from build123d import *

# Parameters (mm, degrees)
SKETCH1_W           = 12.7
SKETCH1_H           = 12.7
BOSS_EXTRUDE1_DEPTH = 2.54
FILLET1_R           = 0.635
SHELL1_START        = 0.635
SHELL1_OUTLINE_W    = 1.905
SHELL1_OUTLINE_H    = 11.43
SHELL1_DEPTH        = 11.43
SKETCH2_R           = 2.54
BOSS_EXTRUDE2_DEPTH = 1.905
BOSS_EXTRUDE3_DEPTH = 0.00254


# Read off the part's stored shape, not the designer's step: Shell1
with BuildPart() as part:
    # Sketch1 → Boss-Extrude1 (new body)
    with BuildSketch(Plane(origin=(0, 0, 0), x_dir=(1, 0, 0), z_dir=(0, 1, 0))):
        with Locations((6.35, 6.35)):
            Rectangle(SKETCH1_W, SKETCH1_H)
    extrude(amount=BOSS_EXTRUDE1_DEPTH)

    # Fillet1
    fillet1_edges = [part.edges().sort_by_distance(p)[0] for p in [
        (0, 1.27, -12.7),
        (12.7, 1.27, -12.7),
        (12.7, 1.27, 0),
        (0, 1.27, 0),
    ]]
    fillet(fillet1_edges, radius=FILLET1_R)

    # Shell1 outline → Shell1 (cut)
    with BuildSketch(Plane.YZ.offset(SHELL1_START)):
        with Locations((0.9525, -6.35)):
            Rectangle(SHELL1_OUTLINE_W, SHELL1_OUTLINE_H)
    extrude(amount=SHELL1_DEPTH, mode=Mode.SUBTRACT)

    # Sketch2 → Boss-Extrude2 (add)
    with BuildSketch(Plane(origin=(0, 1.905, 0), x_dir=(-1, 0, 0), z_dir=(0, -1, 0))):
        with Locations(Location((-6.35, 6.35, 0), (0, 0, 270))):
            Circle(SKETCH2_R)
    extrude(amount=BOSS_EXTRUDE2_DEPTH)

    # Sketch3 → Boss-Extrude3 (add)
    with BuildSketch(Plane(origin=(0, 2.54, 0), x_dir=(1, 0, 0), z_dir=(0, 1, 0))):
        Polygon((4.851562821, 8.001), (5.460231691, 8.001), (6.276242308, 5.74568149), (7.094160978, 8.001), (7.700921795, 8.001), (6.549729888, 4.826), (6.000846675, 4.826), align=None)
    extrude(amount=BOSS_EXTRUDE3_DEPTH)


solid = part.part
Could you check a few things on this model? Use its own coordinates, in mm. A direction names the side the tool comes from. Round coordinates to 2 decimals unless told otherwise and drop trailing zeros. Order: outer loops, then holes, each group sorted by start corner. A loop starts at its lowest first (then second) coordinate and runs counter-clockwise, first axis right, second up.
Q1. Imagine slicing it at A-A, the plane y = 1.35. List the corners of the cut face in (x, z) for me (3 decimals).
Geometry says:
outline: (0, -12.065) arc R0.635 ccw to (0.635, -12.7) - (12.065, -12.7) arc R0.635 ccw to (12.7, -12.065) - (12.7, -0.635) arc R0.635 ccw to (12.065, 0) - (0.635, 0) arc R0.635 ccw to (0, -0.635) - close; circle Ø5.08 at (6.35, -6.35); hole (0.635, -12.065) - (12.065, -12.065) - (12.065, -0.635) - (0.635, -0.635) - close
Q2. Which directions (+Z, -Z, +X, -X, +Y, -Y) give clear straight access to the entire face, cutting with the end or side of a thin tool? Please do faces 1 (the face through (8.83, 0.97, -6.9)), 2 (the face through (6, 2.543, -6)).
Geometry says:
face 1: -Y
face 2: +Z, -Z, +X, -X, +Y
Q3. Imagine slicing it at C-C, the plane z = -9.5. List the corners of the cut face in (x, y) for me (3 decimals).
Geometry says:
outline: (0, 0) - (0.635, 0) - (0.635, 1.905) - (12.065, 1.905) - (12.065, 0) - (12.7, 0) - (12.7, 2.54) - (0, 2.54) - close
Q4. Please list where these lines run through material, in increasing order: probe 1 along X at (y, z) = (1.55, -9.5) (3 decimals); probe 2 along Z at (x, y) = (10.25, 1.7) (3 decimals); probe 3 along Z at (x, y) = (6.25, 1.15) (3 decimals).
Geometry says:
probe 1: x = 0 to 0.635, 12.065 to 12.7
probe 2: z = -12.7 to -12.065, -0.635 to 0
probe 3: z = -12.7 to -12.065, -8.888 to -3.812, -0.635 to 0
Q5. Thinking about a two-plate mould opening in Z: for faces 3 (the face through (6, 1, -12.7)), 4 (the face through (5, 1.905, -9)), 5 (the face through (12.065, 1, -6)), 6 (the face through (5.8, 0, -0.3)), which applies, released by +Z, released by -Z, zero draft, split by the parting line, or undercut?
Geometry says:
face 3: released by -Z
face 4: undercut
face 5: undercut
face 6: zero draft
Q6. Imagine slicing it at B-B, the plane x = 11.5. List the corners of the cut face in (y, z) for me (3 decimals), then the cut area to 3 significant figures.
Geometry says:
outline: (0, -12.7) - (2.54, -12.7) - (2.54, 0) - (0, 0) - (0, -0.635) - (1.905, -0.635) - (1.905, -12.065) - (0, -12.065) - close
area: 10.5 mm2
